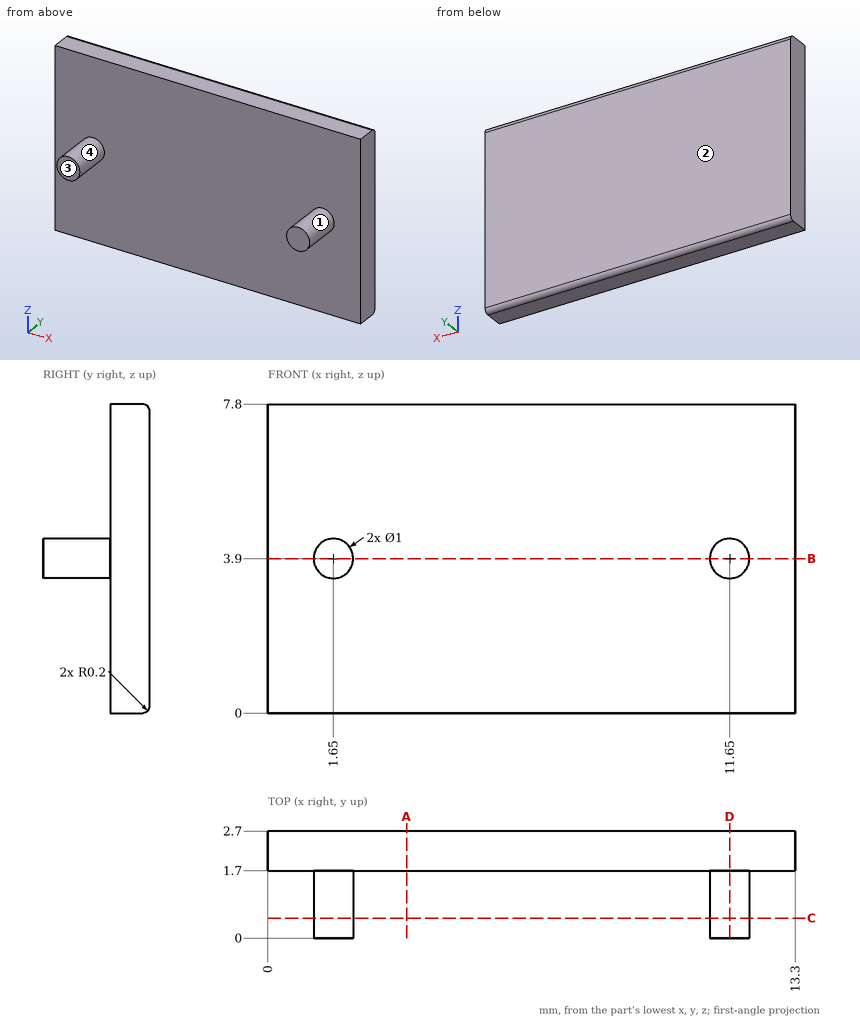
Can you work these out from the drawing? Everything is in mm from the part's minimum corner. A direction names the side the tool comes from. Coordinates: 2 decimals unless noted, no trailing zeros. Loops run counter-clockwise (first coordinate to the right, second up) from the corner with the lowest first, then second, coordinate; pieces in that order, holes last.
1) Which directions (+Z, -Z, +X, -X, +Y, -Y) give clear straight access to the entire face, cutting with the end or side of a thin tool? Please do the marked faces 3 and 4.
2) Imagine slicing it at D-D on x = 11.65. List the corners of the cut face in (y, z) for me.
3) Imagine slicing it at A-A on x = 3.5. List the corners of the cut face in (y, z) for me.
4) Thinking about a two-plate mould opening in X: for the marked faces 1 and 2, which applies, pulls with the +X half, pulls with the -X half, needs draft (parallel to the pull), parting line crosses it, or undercut?
5) Imagine slicing it at B-B on z = 3.9. List the corners of the cut face in (x, y) for me, plus the area to 3 significant figures.
6) Imagine slicing it at C-C on y = 0.5. List the corners of the cut face in (x, z) for me, plus the area to 3 significant figures.
7) I need wall thicknesses on probe 1 along Y at (x, z) = (6, 0.75); probe 2 along X at (y, z) = (0.3, 3.5); probe 3 along Z at (x, y) = (1.25, 0.8). Which ranges of each line are inside material? Lowest first, please.
Completed:
1. face 3: +Z, -Z, +X, -X, -Y
1. face 4: -Y
2. outline: (0, 3.4) - (1.7, 3.4) - (1.7, 0) - (2.5, 0) arc R0.2 ccw to (2.7, 0.2) - (2.7, 7.6) arc R0.2 ccw to (2.5, 7.8) - (1.7, 7.8) - (1.7, 4.4) - (0, 4.4) - close
3. outline: (1.7, 0) - (2.5, 0) arc R0.2 ccw to (2.7, 0.2) - (2.7, 7.6) arc R0.2 ccw to (2.5, 7.8) - (1.7, 7.8) - close
4. face 1: undercut
4. face 2: needs draft
5. outline: (0, 1.7) - (1.15, 1.7) - (1.15, 0) - (2.15, 0) - (2.15, 1.7) - (11.15, 1.7) - (11.15, 0) - (12.15, 0) - (12.15, 1.7) - (13.3, 1.7) - (13.3, 2.7) - (0, 2.7) - close
5. area: 16.7 mm2
6. outline: circle Ø1 at (1.65, 3.9); circle Ø1 at (11.65, 3.9)
6. area: 1.57 mm2
7. probe 1: y = 1.7 to 2.7
7. probe 2: x = 1.35 to 1.95, 11.35 to 11.95
7. probe 3: z = 3.6 to 4.2
